Design review of the part built by this model. Coordinates are the model's own, in mm. A direction names the side the tool comes from. Coordinates: 2 decimals unless noted, no trailing zeros. Loops run counter-clockwise (first coordinate to the right, second up) from the corner with the lowest first, then second, coordinate; pieces in that order, holes last. Notation, with made-up numbers: (42.5, -13) - (64.5, -13) arc R12 cw to (64.5, -8) - close; hole circle Ø5 at (83, -19.75). An arc over 180 degrees is marked (long way). One line per question, with ' | ' between items.
from build123d import *

# Parameters (mm, degrees)
SKETCH_1_R               = 3
EXTRUDE_1_DEPTH          = 180
SKETCH_2_R               = 8
EXTRUDE_2_DEPTH          = 2
EXTRUDE_START            = -178
SKETCH_2_2_R             = 8
EXTRUDE_3_DEPTH          = 2
EXTRUDE_START_2          = -2
SKETCH_1_2_R             = 3
EXTRUDE_4_DEPTH          = 2
EXTRUDE_START_3          = 180
SKETCH_1_3_R             = 3
EXTRUDE_5_DEPTH          = 2
EXTRUDE_START_4          = 4
SKETCH_2_3_R             = 8
EXTRUDE_6_DEPTH          = 2
EXTRUDE_START_5          = -182
SKETCH_2_4_R             = 8
EXTRUDE_7_DEPTH          = 2
EXTRUDE_START_6          = -64
SKETCH_3_R               = 5
EXTRUDE_10_DEPTH         = 60
CUT_EXTRUDE_1_DEPTH      = 185.347497949
CUT_EXTRUDE_1_DEPTH_BACK = 185.347497949
SKETCH_4_W               = 129.449632944
SKETCH_4_H               = 45.19740272
EXTRUDE_START_7          = 20
SKETCH_5_R               = 5
EXTRUDE_11_DEPTH         = 20
EXTRUDE_START_8          = 40
SKETCH_5_2_R             = 5
EXTRUDE_12_DEPTH         = 40


with BuildPart() as part:
    # 草图1 → 凸台-拉伸1 (new body)
    with BuildSketch(Plane.XY):
        with Locations(Location((0, 0, 0), (0, 0, 180))):
            Circle(SKETCH_1_R)
    extrude(amount=EXTRUDE_1_DEPTH)

    # 草图2 → 凸台-拉伸2 (add)
    with BuildSketch(Plane.XY.offset(180)):
        Circle(SKETCH_2_R)
    extrude(amount=-EXTRUDE_2_DEPTH)

    # 草图2<2> → 凸台-拉伸3 (add)
    with BuildSketch(Plane.XY.offset(180).offset(EXTRUDE_START)):
        Circle(SKETCH_2_2_R)
    extrude(amount=-EXTRUDE_3_DEPTH)

    # 草图1<2> → 凸台-拉伸4 (add)
    with BuildSketch(Plane.XY.offset(EXTRUDE_START_2)):
        with Locations(Location((0, 0, 0), (0, 0, 180))):
            Circle(SKETCH_1_2_R)
    extrude(amount=EXTRUDE_4_DEPTH)

    # 草图1<3> → 凸台-拉伸5 (add)
    with BuildSketch(Plane.XY.offset(EXTRUDE_START_3)):
        with Locations(Location((0, 0, 0), (0, 0, 180))):
            Circle(SKETCH_1_3_R)
    extrude(amount=EXTRUDE_5_DEPTH)

    # 草图2<3> → 凸台-拉伸6 (add)
    with BuildSketch(Plane.XY.offset(180).offset(EXTRUDE_START_4)):
        Circle(SKETCH_2_3_R)
    extrude(amount=-EXTRUDE_6_DEPTH)

    # 草图2<4> → 凸台-拉伸7 (add)
    with BuildSketch(Plane.XY.offset(180).offset(EXTRUDE_START_5)):
        Circle(SKETCH_2_4_R)
    extrude(amount=-EXTRUDE_7_DEPTH)

    # 草图3 → 凸台-拉伸10 (add)
    with BuildSketch(Plane.XY.offset(184).offset(EXTRUDE_START_6)):
        Circle(SKETCH_3_R)
    extrude(amount=-EXTRUDE_10_DEPTH)

    # 草图4 → 切除-拉伸1 (cut, two sides: drawn at the far end of the back side and taken through both)
    with BuildSketch(Plane(origin=(0, 0, 0), x_dir=(0, 0, -1), z_dir=(1, 0, 0)).offset(-CUT_EXTRUDE_1_DEPTH_BACK)):
        with Locations((-45.596015123, 0.262013929)):
            Rectangle(SKETCH_4_W, SKETCH_4_H)
    extrude(amount=CUT_EXTRUDE_1_DEPTH + CUT_EXTRUDE_1_DEPTH_BACK, mode=Mode.SUBTRACT)

    # 草图5 → 凸台-拉伸11 (add)
    with BuildSketch(Plane.XY.offset(120).offset(EXTRUDE_START_7)):
        Circle(SKETCH_5_R)
    extrude(amount=-EXTRUDE_11_DEPTH)

    # 草图5<2> → 凸台-拉伸12 (add)
    with BuildSketch(Plane.XY.offset(120).offset(EXTRUDE_START_8)):
        Circle(SKETCH_5_2_R)
    extrude(amount=-EXTRUDE_12_DEPTH)


solid = part.part
Q1. To check wall thickness, follow line 1 along Z through (x, y) = (3.25, -1.25); line 2 along Z through (x, y) = (-7, -3.5); line 3 along X through (y, z) = (-4, 144). State the ranges of each line that lie inside material, in increasing order.
Returned:
line 1: z = 110.32 to 160, 178 to 180, 182 to 184 | line 2: z = 178 to 180, 182 to 184 | line 3: x = -3 to 3
Q2. Draft analysis for pull direction Z (two halves, no side actions). For faces 4 (the cylindrical face through (-1.73, -7.81, 183.01)), 5 (the flat face through (3.4, 0.1, 180)), 6 (the flat face through (0, 0, 110.321)), state which applies: +Z half, -Z half, draft (parallel to the pull), parting line (faces both ways), or undercut.
Returned:
face 4: draft | face 5: undercut | face 6: -Z half
Q3. Take a section at D-D (y = 4). Give the boundary of the cut face in (x, z).
Returned:
outline: (-6.93, 178) - (6.93, 178) - (6.93, 180) - (-6.93, 180) - close; (-6.93, 182) - (6.93, 182) - (6.93, 184) - (-6.93, 184) - close; (-3, 110.32) - (3, 110.32) - (3, 160) - (-3, 160) - close
Q4. Tool access review of faces 1 (the cylindrical face through (-1.08, -4.88, 135.51)), 2 (the flat face through (-0.1, -3.3, 160)), 3 (the cylindrical face through (-1.73, -7.81, 179.01)): name each direction out of +Z, -Z, +X, -X, +Y, -Y from which nothing blocks a thin tool from reaching the whole face with its end or side.
Returned:
face 1: -Z | face 2: none | face 3: +Z, -Z
Q5. For pin 1 (8 mm diameter, centred on y = 1.5, z = 173, fed in from +X); pin 2 (6 mm diameter, centred on x = -1, y = 5.5, fed in from -Z); pin 3 (6 mm diameter, centred on y = 1.5, z = 147, fed in from +X); pin 4 (1 mm diameter, centred on x = 3, z = 148.5, fed in from +Y), all flat-tipped, find the tip position at first contact; note any pin that passes through.
Returned:
pin 1: stops at x = 3 | pin 2: stops at z = 110.32 | pin 3: stops at x = 5 | pin 4: stops at y = 4.33
Q6. Take a section at A-A (y = 0). Give the boundary of the cut face in (x, z).
Returned:
outline: (-8, 178) - (-3, 178) - (-3, 160) - (-5, 160) - (-5, 110.32) - (5, 110.32) - (5, 160) - (3, 160) - (3, 178) - (8, 178) - (8, 180) - (3, 180) - (3, 182) - (8, 182) - (8, 184) - (-8, 184) - (-8, 182) - (-3, 182) - (-3, 180) - (-8, 180) - close
Q7. Take a section at C-C (y = 7). Give the boundary of the cut face in (x, z).
Returned:
outline: (-3.87, 178) - (3.87, 178) - (3.87, 180) - (-3.87, 180) - close; (-3.87, 182) - (3.87, 182) - (3.87, 184) - (-3.87, 184) - close
